```python
from build123d import *


with BuildPart() as part:
    # Sketch1 → Revolve1 (revolve)
    with BuildSketch(Plane(origin=(0, 0, 0), x_dir=(0, 0, -1), z_dir=(1, 0, 0))):
        with BuildLine():
            Line((0, 0), (17, 0))
            ThreePointArc((17, 0), (27.606601718, 4.393398282), (32, 15))
            Line((32, 15), (32, 114.751276219))
            ThreePointArc((32, 114.751276219), (31.652603278, 118.46276977), (30.622481562, 122.045327253))
            Line((30.622481562, 122.045327253), (16.377518438, 158.414220463))
            ThreePointArc((16.377518438, 158.414220463), (15.347396722, 161.996777946), (15, 165.708271497))
            Line((15, 165.708271497), (15, 221.5))
            ThreePointArc((15, 221.5), (14.853553391, 221.853553391), (14.5, 222))
            Line((14.5, 222), (13, 222))
            ThreePointArc((13, 222), (12.646446609, 221.853553391), (12.5, 221.5))
            Line((12.5, 221.5), (12.5, 211.633388036))
            Line((12.5, 211.633388036), (12.5, 165.23613385))
            ThreePointArc((12.5, 165.23613385), (12.847396722, 161.524640298), (13.877518438, 157.942082816))
            Line((13.877518438, 157.942082816), (28.122481562, 121.573189605))
            ThreePointArc((28.122481562, 121.573189605), (29.152603278, 117.990632123), (29.5, 114.279138571))
            Line((29.5, 114.279138571), (29.5, 17.5))
            ThreePointArc((29.5, 17.5), (25.106601718, 6.893398282), (14.5, 2.5))
            Line((14.5, 2.5), (0, 2.5))
            Line((0, 2.5), (0, 0))
        make_face()
    revolve(axis=Axis((0, 0, 0), (0, 1, 0)))


solid = part.part
```
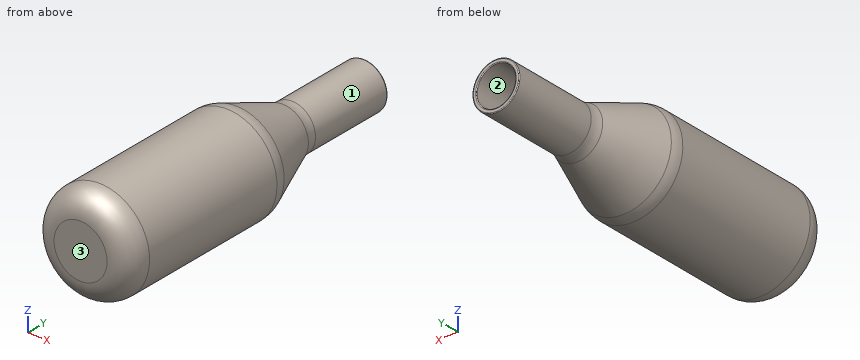
The model under review builds one solid part; all positions refer to its coordinate system, in mm. Face numbers are marked on the shaded views. Round coordinates to 2 decimals unless told otherwise and drop trailing zeros. Write each loop counter-clockwise with the first axis right and the second up, starting at its lowest first coordinate (ties: lowest second). Pieces come first, ordered by that corner, then holes. Notation, with made-up numbers: M 65.5,19 L 115.5,19 A25 ccw 115.5,45 Z; hole C 3,30 d2. An arc over 180 degrees is marked long. Use CSV: the item, a comma, the result in double quotes. Start each with the question number.
(1) Clearance check with flat-ended pins moving along their axes: P1, Ø6, axis at y = 65.5, z = 13, coming from the +X side; P2, Ø12, axis at y = 141.5, z = -12, coming from the +X side; P3, Ø1, axis at y = 155, z = 14, coming from the +X side. State where each tip first meets the part, or that it passes through.
(2) The part is to be moulded in two halves that separate along X. For the marked faces 1, 2 and 3, say which applies: +X half, -X half, draft (parallel to the pull), parting line (faces both ways), or undercut.
(3) For line 1 along X through (y, z) = (50.5, 0); line 2 along X through (y, z) = (204.5, 0), list the stretches that pass through material, from the lowest coordinate up.
(4) We need section B-B, the plane y = 25.5. State the section outline as (x, z) points, then the cut area to 3 significant figures.
(5) We need section A-A, the plane y = 180.5. State the section outline as (x, z) points, then the cut area to 3 significant figures.
Findings:
1,P1,"x = 30.4"
1,P2,"x = 23.43"
1,P3,"x = 11.54"
2,face 1,"parting line"
2,face 2,"undercut"
2,face 3,"draft"
3,line 1,"-32 to -29.5, 29.5 to 32"
3,line 2,"-15 to -12.5, 12.5 to 15"
4,outline,"C 0,0 d64; hole C 0,0 d59"
4,area,"483 mm^2"
5,outline,"C 0,0 d30; hole C 0,0 d25"
5,area,"216 mm^2"
